```python
from build123d import *

# Parameters (mm, degrees)
EXTRUSION1_DEPTH        = 130
PER_AGE1_OUTLINE_R      = 2.1
PER_AGE1_DEPTH          = 130
ENL_V_MAT_EXTRU_1_DEPTH = 300
ENL_V_MAT_EXTRU_3_DEPTH = 300
ENL_V_MAT_EXTRU_4_DEPTH = 131.766968306
ENL_V_MAT_EXTRU_7_DEPTH = 131.766968306


# Read off the part's stored shape, not the designer's step: Perçage1
with BuildPart() as part:
    # Esquisse1 → Extrusion1 (new body)
    with BuildSketch(Plane.XY):
        with BuildLine():
            Line((-10, 8), (-10, -8))
            ThreePointArc((-10, -8), (-9.414213562, -9.414213562), (-8, -10))
            Line((-8, -10), (8, -10))
            ThreePointArc((8, -10), (9.414213562, -9.414213562), (10, -8))
            Line((10, -8), (10, 8))
            ThreePointArc((10, 8), (9.414213562, 9.414213562), (8, 10))
            Line((8, 10), (-8, 10))
            ThreePointArc((-8, 10), (-9.414213562, 9.414213562), (-10, 8))
        make_face()
    extrude(amount=EXTRUSION1_DEPTH)

    # Perçage1 outline → Perçage1 (cut)
    with BuildSketch(Plane.XY):
        Circle(PER_AGE1_OUTLINE_R)
    extrude(amount=PER_AGE1_DEPTH, mode=Mode.SUBTRACT)

    # Esquisse3 → Enlèv. mat.-Extru.1 (cut)
    with BuildSketch(Plane.XY.offset(130)):
        Polygon((10, 2.5), (8.2, 2.5), (8.2, 6), (3.7, 2.5), (3.7, -2.5), (8.2, -6), (8.2, -2.5), (10, -2.5), align=None)
    extrude(amount=-ENL_V_MAT_EXTRU_1_DEPTH, mode=Mode.SUBTRACT)

    # Esquisse5 → Enlèv. mat.-Extru.3 (cut)
    with BuildSketch(Plane.XY.offset(130)):
        Polygon((-2.5, 10), (-2.5, 8.2), (-6, 8.2), (-2.5, 3.7), (2.5, 3.7), (6, 8.2), (2.5, 8.2), (2.5, 10), align=None)
    extrude(amount=-ENL_V_MAT_EXTRU_3_DEPTH, mode=Mode.SUBTRACT)

    # Esquisse6 → Enlèv. mat.-Extru.4 (cut, through all)
    with BuildSketch(Plane.XY.offset(130)):
        Polygon((-2.5, -10), (-2.5, -8.2), (-6, -8.2), (-2.5, -3.7), (2.5, -3.7), (6, -8.2), (2.5, -8.2), (2.5, -10), align=None)
    extrude(amount=-ENL_V_MAT_EXTRU_4_DEPTH, mode=Mode.SUBTRACT)

    # Esquisse4 → Enlèv. mat.-Extru.7 (cut, through all)
    with BuildSketch(Plane.XY.offset(130)):
        Polygon((-10, 2.5), (-8.2, 2.5), (-8.2, 6), (-3.7, 2.5), (-3.7, -2.5), (-8.2, -6), (-8.2, -2.5), (-10, -2.5), align=None)
    extrude(amount=-ENL_V_MAT_EXTRU_7_DEPTH, mode=Mode.SUBTRACT)


solid = part.part
```
For this review, take the finished solid that the model builds, in its own axes (mm). A direction names the side the tool comes from. Round coordinates to 2 decimals unless told otherwise and drop trailing zeros. Write each loop counter-clockwise with the first axis right and the second up, starting at its lowest first coordinate (ties: lowest second). Pieces come first, ordered by that corner, then holes. Notation, with made-up numbers: (71, 83.5) - (102, 83.5) arc R17 cw to (102, 102.5) - close; hole circle Ø6 at (-15.75, -8.5). An arc over 180 degrees is marked (long way). Put each result on its own line as item: value.
Q1. Insertion check: pin 1 Ø0.5 at (y, z) = (-9.5, 52) entering from -X; pin 2 Ø2 at (x, z) = (0, 108) entering from -Y; pin 3 Ø0.9 at (x, z) = (9, 85) entering from +Y. Each pin has a flat end and moves straight along its axis. Give the tip position at first contact, or say it passes through.
Solved:
pin 1: stops at x = -9.56
pin 2: stops at y = -3.7
pin 3: stops at y = 9.92
Q2. Mouldability with a two-part tool opening along Y and no side actions: class faces 4 (the face through (5, -10, 64)), 5 (the face through (-0.1, 2.4, 0)), 6 (the face through (0, 3.7, 66)), 7 (the face through (5.919, -4.226, 65.91)) as released by +Y, released by -Y, zero draft, split by the parting line, or undercut.
Solved:
face 4: released by -Y
face 5: zero draft
face 6: released by +Y
face 7: undercut
Q3. Machinability: for faces 1 (the face through (0, -3.7, 66)), 2 (the face through (9.4, -9.43, 64.09)), 3 (the face through (-3.7, 0, 66)), which of the approach directions +Z, -Z, +X, -X, +Y, -Y give a long, thin tool a straight path to every point of the face, cutting with its end or side? Answer none if there is none.
Solved:
face 1: +Z, -Z, -Y
face 2: +Z, -Z, +X, -Y
face 3: +Z, -Z, -X
Q4. We need section A-A (x = 0). Give the boundary of the cut face in (y, z).
Solved:
outline: (-3.7, 0) - (-2.1, 0) - (-2.1, 130) - (-3.7, 130) - close; (2.1, 0) - (3.7, 0) - (3.7, 130) - (2.1, 130) - close
Q5. Wall thickness on probe 1 along Y at (x, z) = (0, 67); probe 2 along X at (y, z) = (-3, 42.5); probe 3 along Y at (x, z) = (-4.25, 77): over which ranges is each line inside the solid? List them lowest first.
Solved:
probe 1: y = -3.7 to -2.1, 2.1 to 3.7
probe 2: x = -10 to -8.2, -4.34 to 4.34, 8.2 to 10
probe 3: y = -10 to -8.2, -5.95 to -2.93, 2.93 to 5.95, 8.2 to 10
